Design review of the part built by this model. Coordinates are the model's own, in mm. Face numbers are marked on the shaded views. A direction names the side the tool comes from. Round coordinates to 2 decimals unless told otherwise and drop trailing zeros. Loops run counter-clockwise (first coordinate to the right, second up) from the corner with the lowest first, then second, coordinate; pieces in that order, holes last. Notation, with made-up numbers: (-36.5, 87) -> (-14.5, 87) arc R22 cw to (-14.5, 108) -> close; hole circle Ø1 at (80, 4.25). An arc over 180 degrees is marked (long way). Write each question's results on one line, items separated by ' | '. Start each with the question number.
from build123d import *

# Parameters (mm, degrees)
SKETCH_1_R      = 11
EXTRUDE_4_DEPTH = 75
EXTRUDE_5_DEPTH = 20
CHAMFER_2_SIZE  = 3


with BuildPart() as part:
    # Эскиз1 → Бобышка-Вытянуть4 (new body)
    with BuildSketch(Plane(origin=(0, 0, 0), x_dir=(1, 0, 0), z_dir=(0, 1, 0))):
        Circle(SKETCH_1_R)
    extrude(amount=EXTRUDE_4_DEPTH)

    # Эскиз3 → Бобышка-Вытянуть5 (add)
    with BuildSketch(Plane.XZ):
        Polygon((0.259699185, 20.035631897), (-17.060808891, 10.035631897), (-17.060808891, -9.964368103), (0.259699185, -19.964368103), (17.58020726, -9.964368103), (17.58020726, 10.035631897), align=None)
    extrude(amount=EXTRUDE_5_DEPTH)

    # Фаска2
    chamfer_2_edges = [part.edges().sort_by_distance(p)[0] for p in [
        (8.919953222, -20, 15.035631897),
        (-8.400554853, -20, 15.035631897),
        (-17.060808891, -20, 0.035631897),
        (-8.400554853, -20, -14.964368103),
        (8.919953222, -20, -14.964368103),
        (17.58020726, -20, 0.035631897),
    ]]
    chamfer(chamfer_2_edges, length=CHAMFER_2_SIZE)


solid = part.part
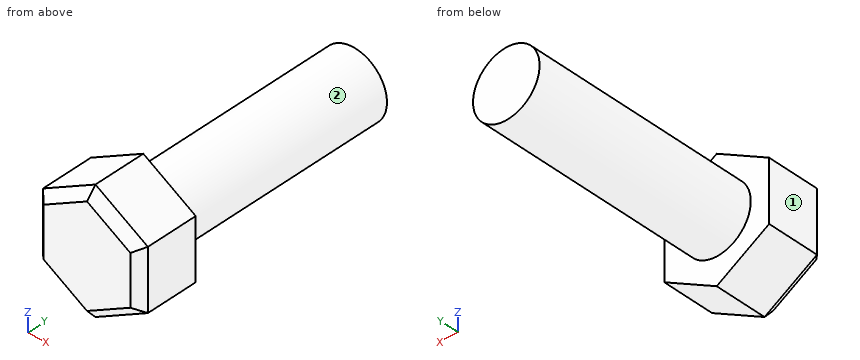
1) To check wall thickness, follow line 1 (Y direction, x = -8.5, z = -11); line 2 (Y direction, x = 10.5, z = -14); line 3 (X direction, y = 10, z = 4.5). State the ranges of each line that lie inside material, in increasing order. Write a range as from..to.
2) For the marked faces 1 and 2, list the 3-axis set-ups (+Z, -Z, +X, -X, +Y, -Y) from which the entire face can be reached by the end or side of a thin tool; tool diameter is ignored.
3) Take a section at A-A (z = 0). Write out the cut boundary in (x, y).
4) Take a section at B-B (y = -3). Write out the cut boundary in (x, z), plus the area to 3 significant figures.
5) Take a section at D-D (y = 58.5). Write out the cut boundary in (x, z), plus the area to 3 significant figures.
6) Take a section at C-C (x = -9). Write out the cut boundary in (y, z).
7) Insertion check: pin 1 (6 mm diameter, centred on x = 5, z = -15.5, fed in from +Y); pin 2 (2 mm diameter, centred on x = 2, y = 26.5, fed in from +Z); pin 3 (6 mm diameter, centred on x = -0.5, y = 38, fed in from -Z). Each pin has a flat end and moves straight along its axis. Give the tip position at first contact, or say it passes through.
Geometry check:
1) line 1: y = -20..0 | line 2: y = -17.05..0 | line 3: x = -10.04..10.04
2) face 1: +Z, -Z, -X, +Y, -Y | face 2: +Y
3) outline: (-17.06, -17) -> (-14.06, -20) -> (14.58, -20) -> (17.58, -17) -> (17.58, 0) -> (11, 0) -> (11, 75) -> (-11, 75) -> (-11, 0) -> (-17.06, 0) -> close
4) outline: (-17.06, -9.96) -> (0.26, -19.96) -> (17.58, -9.96) -> (17.58, 10.04) -> (0.26, 20.04) -> (-17.06, 10.04) -> close | area: 1,040 mm^2
5) outline: circle Ø22 at (0, 0) | area: 380 mm^2
6) outline: (-20, -11.15) -> (-17, -14.62) -> (0, -14.62) -> (0, -6.32) -> (75, -6.32) -> (75, 6.32) -> (0, 6.32) -> (0, 14.69) -> (-17, 14.69) -> (-20, 11.23) -> close
7) pin 1: stops at y = 0 | pin 2: stops at z = 10.95 | pin 3: stops at z = -11
